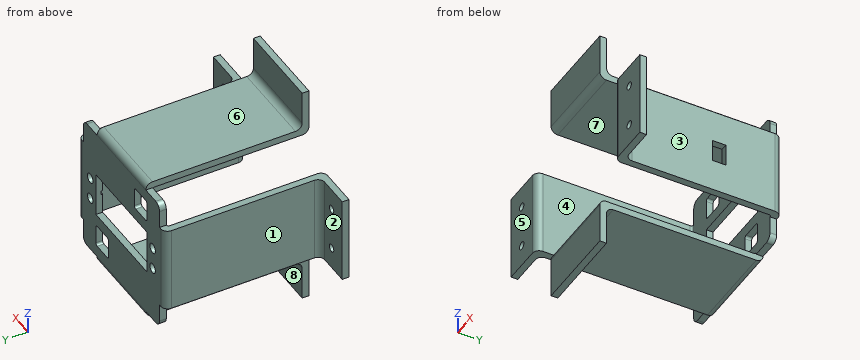
```python
from build123d import *

# Parameters (mm, degrees)
SALIENTE_EXTRUIR1_DEPTH = 19.5
CROQUIS1_4_W            = 30.5
CROQUIS1_4_H            = 3
SALIENTE_EXTRUIR2_DEPTH = 30.5
CORTAR_EXTRUIR1_REACH   = 96.401
CROQUIS2_R              = 2.2
CROQUIS2_W              = 40.8
CROQUIS2_H              = 20
CROQUIS2_W_2            = 10
CROQUIS2_H_2            = 10
CROQUIS3_W              = 7
CROQUIS3_H              = 1.8
CORTAR_EXTRUIR2_DEPTH   = 0.8
CORTAR_EXTRUIR3_REACH   = 96.401
CROQUIS4_R              = 1.75
REDONDEO1_R             = 3
REDONDEO2_R             = 1
SALIENTE_EXTRUIR3_DEPTH = 19.5
REDONDEO3_R             = 3
REDONDEO4_R             = 1
CROQUIS10_W             = 10
CROQUIS10_H             = 6
CORTAR_EXTRUIR4_DEPTH   = 122.94363452


with BuildPart() as part:
    # Croquis1 → Saliente-Extruir1 (new, symmetric)
    with BuildSketch(Plane.XY):
        Polygon((-51.5, 0), (-31.5, 0), (-31.5, 70), (31.5, 70), (31.5, 0), (51.5, 0), (51.5, 3), (34.5, 3), (34.5, 73), (-34.5, 73), (-34.5, 3), (-51.5, 3), align=None)
    extrude(amount=SALIENTE_EXTRUIR1_DEPTH, both=True)

    # Croquis1_4 → Saliente-Extruir2 (add, symmetric)
    with BuildSketch(Plane.XY):
        with Locations((-15.25, 71.5)):
            Rectangle(CROQUIS1_4_W, CROQUIS1_4_H)
        with Locations((15.25, 71.5)):
            Rectangle(CROQUIS1_4_W, CROQUIS1_4_H)
    extrude(amount=SALIENTE_EXTRUIR2_DEPTH, both=True)

    # Croquis2 → Cortar-Extruir1 (cut, up to next)
    with BuildSketch(Plane(origin=(0, 73, 0), x_dir=(1, 0, 0), z_dir=(0, 1, 0)), mode=Mode.PRIVATE) as cortar_extruir1_sk1:
        with Locations(Location((24.97, 5, 0), (0, 0, 270))):
            Circle(CROQUIS2_R)
    cortar_extruir1_tool1 = extrude(cortar_extruir1_sk1.sketch, amount=-CORTAR_EXTRUIR1_REACH, mode=Mode.PRIVATE) & part.part
    # Croquis2 → Cortar-Extruir1 (cut, up to next)
    with BuildSketch(Plane(origin=(0, 73, 0), x_dir=(1, 0, 0), z_dir=(0, 1, 0)), mode=Mode.PRIVATE) as cortar_extruir1_sk2:
        with Locations(Location((24.97, -5, 0), (0, 0, 270))):
            Circle(CROQUIS2_R)
    cortar_extruir1_tool2 = extrude(cortar_extruir1_sk2.sketch, amount=-CORTAR_EXTRUIR1_REACH, mode=Mode.PRIVATE) & part.part
    # Croquis2 → Cortar-Extruir1 (cut, up to next)
    with BuildSketch(Plane(origin=(0, 73, 0), x_dir=(1, 0, 0), z_dir=(0, 1, 0)), mode=Mode.PRIVATE) as cortar_extruir1_sk3:
        with Locations(Location((-24.97, 5, 0), (0, 0, 270))):
            Circle(CROQUIS2_R)
    cortar_extruir1_tool3 = extrude(cortar_extruir1_sk3.sketch, amount=-CORTAR_EXTRUIR1_REACH, mode=Mode.PRIVATE) & part.part
    # Croquis2 → Cortar-Extruir1 (cut, up to next)
    with BuildSketch(Plane(origin=(0, 73, 0), x_dir=(1, 0, 0), z_dir=(0, 1, 0)), mode=Mode.PRIVATE) as cortar_extruir1_sk4:
        with Locations(Location((-24.97, -5, 0), (0, 0, 270))):
            Circle(CROQUIS2_R)
    cortar_extruir1_tool4 = extrude(cortar_extruir1_sk4.sketch, amount=-CORTAR_EXTRUIR1_REACH, mode=Mode.PRIVATE) & part.part
    # Croquis2 → Cortar-Extruir1 (cut, up to next)
    with BuildSketch(Plane(origin=(0, 73, 0), x_dir=(1, 0, 0), z_dir=(0, 1, 0)), mode=Mode.PRIVATE) as cortar_extruir1_sk5:
        Rectangle(CROQUIS2_W, CROQUIS2_H)
    cortar_extruir1_tool5 = extrude(cortar_extruir1_sk5.sketch, amount=-CORTAR_EXTRUIR1_REACH, mode=Mode.PRIVATE) & part.part
    # Croquis2 → Cortar-Extruir1 (cut, up to next)
    with BuildSketch(Plane(origin=(0, 73, 0), x_dir=(1, 0, 0), z_dir=(0, 1, 0)), mode=Mode.PRIVATE) as cortar_extruir1_sk6:
        with Locations((15.4, 20.25)):
            Rectangle(CROQUIS2_W_2, CROQUIS2_H_2)
    cortar_extruir1_tool6 = extrude(cortar_extruir1_sk6.sketch, amount=-CORTAR_EXTRUIR1_REACH, mode=Mode.PRIVATE) & part.part
    # Croquis2 → Cortar-Extruir1 (cut, up to next)
    with BuildSketch(Plane(origin=(0, 73, 0), x_dir=(1, 0, 0), z_dir=(0, 1, 0)), mode=Mode.PRIVATE) as cortar_extruir1_sk7:
        with Locations((-15.4, -20.25)):
            Rectangle(CROQUIS2_W_2, CROQUIS2_H_2)
    cortar_extruir1_tool7 = extrude(cortar_extruir1_sk7.sketch, amount=-CORTAR_EXTRUIR1_REACH, mode=Mode.PRIVATE) & part.part
    add(cortar_extruir1_tool1.solids().sort_by_distance((24.97, 73, -5))[0], mode=Mode.SUBTRACT)
    add(cortar_extruir1_tool2.solids().sort_by_distance((24.97, 73, 5))[0], mode=Mode.SUBTRACT)
    add(cortar_extruir1_tool3.solids().sort_by_distance((-24.97, 73, -5))[0], mode=Mode.SUBTRACT)
    add(cortar_extruir1_tool4.solids().sort_by_distance((-24.97, 73, 5))[0], mode=Mode.SUBTRACT)
    add(cortar_extruir1_tool5.solids().sort_by_distance((0, 73, 0))[0], mode=Mode.SUBTRACT)
    add(cortar_extruir1_tool6.solids().sort_by_distance((15.4, 73, -20.25))[0], mode=Mode.SUBTRACT)
    add(cortar_extruir1_tool7.solids().sort_by_distance((-15.4, 73, 20.25))[0], mode=Mode.SUBTRACT)

    # Croquis3 → Cortar-Extruir2 (cut)
    with BuildSketch(Plane.XZ.offset(-70)):
        with Locations((23.9, 0)):
            Rectangle(CROQUIS3_W, CROQUIS3_H)
        with Locations((-23.9, 0)):
            Rectangle(CROQUIS3_W, CROQUIS3_H)
    extrude(amount=-CORTAR_EXTRUIR2_DEPTH, mode=Mode.SUBTRACT)

    # Croquis4 → Cortar-Extruir3 (cut, up to next)
    with BuildSketch(Plane.XZ, mode=Mode.PRIVATE) as cortar_extruir3_sk1:
        with Locations(Location((43, 9.75, 0), (0, 0, 270))):
            Circle(CROQUIS4_R)
    cortar_extruir3_tool1 = extrude(cortar_extruir3_sk1.sketch, amount=-CORTAR_EXTRUIR3_REACH, mode=Mode.PRIVATE) & part.part
    # Croquis4 → Cortar-Extruir3 (cut, up to next)
    with BuildSketch(Plane.XZ, mode=Mode.PRIVATE) as cortar_extruir3_sk2:
        with Locations(Location((43, -9.75, 0), (0, 0, 270))):
            Circle(CROQUIS4_R)
    cortar_extruir3_tool2 = extrude(cortar_extruir3_sk2.sketch, amount=-CORTAR_EXTRUIR3_REACH, mode=Mode.PRIVATE) & part.part
    # Croquis4 → Cortar-Extruir3 (cut, up to next)
    with BuildSketch(Plane.XZ, mode=Mode.PRIVATE) as cortar_extruir3_sk3:
        with Locations(Location((-43, -9.75, 0), (0, 0, 270))):
            Circle(CROQUIS4_R)
    cortar_extruir3_tool3 = extrude(cortar_extruir3_sk3.sketch, amount=-CORTAR_EXTRUIR3_REACH, mode=Mode.PRIVATE) & part.part
    # Croquis4 → Cortar-Extruir3 (cut, up to next)
    with BuildSketch(Plane.XZ, mode=Mode.PRIVATE) as cortar_extruir3_sk4:
        with Locations(Location((-43, 9.75, 0), (0, 0, 270))):
            Circle(CROQUIS4_R)
    cortar_extruir3_tool4 = extrude(cortar_extruir3_sk4.sketch, amount=-CORTAR_EXTRUIR3_REACH, mode=Mode.PRIVATE) & part.part
    add(cortar_extruir3_tool1.solids().sort_by_distance((43, 0, 9.75))[0], mode=Mode.SUBTRACT)
    add(cortar_extruir3_tool2.solids().sort_by_distance((43, 0, -9.75))[0], mode=Mode.SUBTRACT)
    add(cortar_extruir3_tool3.solids().sort_by_distance((-43, 0, -9.75))[0], mode=Mode.SUBTRACT)
    add(cortar_extruir3_tool4.solids().sort_by_distance((-43, 0, 9.75))[0], mode=Mode.SUBTRACT)

    # Redondeo1
    redondeo1_edges = [part.edges().sort_by_distance(p)[0] for p in [
        (-31.5, 0, 0),
        (-34.5, 3, 0),
        (-34.5, 73, 0),
        (34.5, 73, 0),
        (34.5, 3, 0),
        (31.5, 0, 0),
        (-30.5, 71.5, 30.5),
        (30.5, 71.5, -30.5),
        (30.5, 71.5, 30.5),
        (-30.5, 71.5, -30.5),
    ]]
    fillet(redondeo1_edges, radius=REDONDEO1_R)

    # Redondeo2
    redondeo2_edges = [part.edges().sort_by_distance(p)[0] for p in [
        (-31.5, 70, 0),
        (31.5, 70, 0),
        (-20.4, 71.5, 25.25),
        (-20.4, 71.5, 15.25),
        (-10.4, 71.5, 15.25),
        (-10.4, 71.5, 25.25),
        (20.4, 71.5, -15.25),
        (10.4, 71.5, -15.25),
        (10.4, 71.5, -25.25),
        (20.4, 71.5, -25.25),
    ]]
    fillet(redondeo2_edges, radius=REDONDEO2_R)

    # Croquis8 → Saliente-Extruir3 (add, symmetric)
    with BuildSketch(Plane(origin=(0, 0, 0), x_dir=(0, 0, -1), z_dir=(1, 0, 0))):
        Polygon((-30.5, 73), (-33.5, 73), (-33.5, 3), (-51.5, 3), (-51.5, 0), (-30.5, 0), (-30.5, 70), align=None)
        Polygon((51.5, 3), (51.5, 0), (30.5, 0), (30.5, 70), (30.5, 73), (33.5, 73), (33.5, 3), align=None)
    extrude(amount=SALIENTE_EXTRUIR3_DEPTH, both=True)

    # Redondeo3
    redondeo3_edges = [part.edges().sort_by_distance(p)[0] for p in [
        (0, 73, -33.5),
        (0, 3, -33.5),
        (0, 0, -30.5),
        (0, 0, 30.5),
        (0, 3, 33.5),
        (0, 73, 33.5),
    ]]
    fillet(redondeo3_edges, radius=REDONDEO3_R)

    # Redondeo4
    redondeo4_edges = [part.edges().sort_by_distance(p)[0] for p in [
        (0, 70, 30.5),
        (0, 70, -30.5),
    ]]
    fillet(redondeo4_edges, radius=REDONDEO4_R)

    # Croquis10 → Cortar-Extruir4 (cut, through all)
    with BuildSketch(Plane(origin=(-31.5, 0, 0), x_dir=(0, 0, -1), z_dir=(1, 0, 0))):
        with Locations((0, 45)):
            Rectangle(CROQUIS10_W, CROQUIS10_H)
    extrude(amount=CORTAR_EXTRUIR4_DEPTH, mode=Mode.SUBTRACT)


solid = part.part
```
Work out the finished part from the listing and answer in its coordinate system (mm). Face numbers are marked on the shaded views. A direction names the side the tool comes from. Coordinates: 2 decimals unless noted, no trailing zeros. Loops run counter-clockwise (first coordinate to the right, second up) from the corner with the lowest first, then second, coordinate; pieces in that order, holes last. Notation, with made-up numbers: (30, 67) - (78, 67) arc R13 cw to (78, 82) - close; hole circle Ø10 at (3, 87). An arc over 180 degrees is marked (long way). Use a Markdown table: item, result.
Item 1: Find section C-C, the plane x = 43. Determine the outline of the cut face in (y, z), and give its area (3 significant figures).
Evaluation:
| item | result |
|---|---|
| outline | (0, -19.5) - (3, -19.5) - (3, -11.5) - (0, -11.5) - close; (0, -8) - (3, -8) - (3, 8) - (0, 8) - close; (0, 11.5) - (3, 11.5) - (3, 19.5) - (0, 19.5) - close |
| area | 96.0 mm2 |
Item 2: The mould has two halves that part along X. Classify the marked faces 1, 2, 3 and 4: +X half, -X half, draft (parallel to the pull), parting line (faces both ways), or undercut.
Evaluation:
| item | result |
|---|---|
| face 1 | -X half |
| face 2 | draft |
| face 3 | +X half |
| face 4 | undercut |
Item 3: Find section A-A, the plane y = 27.5. Determine the outline of the cut face in (x, z), and give its area (3 significant figures).
Evaluation:
| item | result |
|---|---|
| outline | (-34.5, -19.5) - (-31.5, -19.5) - (-31.5, 19.5) - (-34.5, 19.5) - close; (-19.5, -33.5) - (19.5, -33.5) - (19.5, -30.5) - (-19.5, -30.5) - close; (-19.5, 30.5) - (19.5, 30.5) - (19.5, 33.5) - (-19.5, 33.5) - close; (31.5, -19.5) - (34.5, -19.5) - (34.5, 19.5) - (31.5, 19.5) - close |
| area | 468 mm2 |
Item 4: Consider probe 1 along Z at (x, y) = (16, 17.5); probe 2 along X at (y, z) = (22.5, 9.5); probe 3 along X at (y, z) = (71, -5). Determine where each line is inside the solid, lowest interval first. Write a range as from..to.
Evaluation:
| item | result |
|---|---|
| probe 1 | z = -33.5..-30.5, 30.5..33.5 |
| probe 2 | x = -34.5..-31.5, 31.5..34.5 |
| probe 3 | x = -34.33..-27.17, -22.77..-20.4, 20.4..22.77, 27.17..34.33 |
Item 5: Find section D-D, the plane z = 44. Determine the outline of the cut face in (x, y), and give its area (3 significant figures).
Evaluation:
| item | result |
|---|---|
| outline | (-19.5, 0) - (19.5, 0) - (19.5, 3) - (-19.5, 3) - close |
| area | 117 mm2 |
Item 6: Given pin 1 Ø19.5 at (y, z) = (47.5, 7) entering from -X; pin 2 Ø11.5 at (y, z) = (44.5, -2.5) entering from +X; pin 3 Ø12 at (x, z) = (-5, 9) entering from -Y, each flat-ended and moving along its own axis, determine where each tip first touches the part or whether it passes through.
Evaluation:
| item | result |
|---|---|
| pin 1 | stops at x = -34.5 |
| pin 2 | stops at x = 34.5 |
| pin 3 | stops at y = 70 |
Item 7: For the marked faces 5, 6, 7 and 8, determine the directions among +Z, -Z, +X, -X, +Y, -Y from which every point of the face is accessible in a straight line to the end or side of a thin tool.
Evaluation:
| item | result |
|---|---|
| face 5 | +Z, -Z, +X, -X, -Y |
| face 6 | +Z, +X, -X, +Y |
| face 7 | +X, -X, -Y |
| face 8 | -Z, +X, -X, +Y |
Item 8: Find section B-B, the plane x = -24.97. Determine the outline of the cut face in (y, z).
Evaluation:
| item | result |
|---|---|
| outline | (70, -30.5) - (73, -30.5) - (73, -7.2) - (70, -7.2) - close; (70, -2.8) - (73, -2.8) - (73, 2.8) - (70, 2.8) - (70, 0.9) - (70.8, 0.9) - (70.8, -0.9) - (70, -0.9) - close; (70, 7.2) - (73, 7.2) - (73, 30.5) - (70, 30.5) - close |
